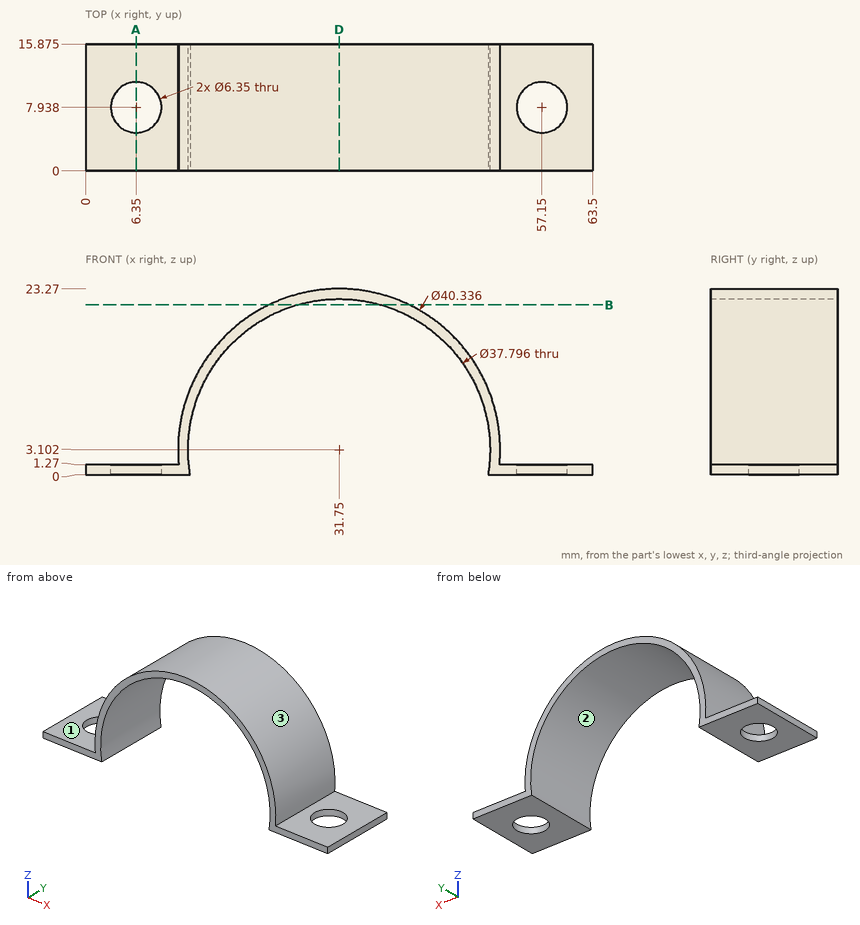
Source: three-view drawing plus pictorial views. Frame: mm from the lowest corner of the part. Coordinates: 2 decimals unless noted, no trailing zeros. Loops run counter-clockwise (first coordinate to the right, second up) from the corner with the lowest first, then second, coordinate; pieces in that order, holes last. Notation, with made-up numbers: (-5.75, 37) -> (29.25, 37) arc R33 cw to (29.25, 76) -> close; hole circle Ø1 at (69, 58). An arc over 180 degrees is marked (long way). Answer in a Markdown table with one row per item. Add a question column.
Q1. Section D-D on x = 31.75. Return the cut outline in (y, z) (1 decimal).
Q2. Section A-A on x = 6.35. Return the cut outline in (y, z) (1 decimal).
Q3. Contact query for flat-ended pins moving along their axis: pin 1 Ø2 at (x, z) = (42.5, 17) entering from +Y; pin 2 Ø6 at (x, y) = (19, 7) entering from +Z; pin 3 Ø6 at (y, z) = (8, 6.5) entering from +X; pin 4 Ø3.5 at (x, y) = (3, 9) entering from +Z. Output: stop coordinate, or through.
Q4. Ray query, line 1 along Y through (x, z) = (6.35, 0.4) (1 decimal); line 2 along Z through (x, y) = (6.5, 1.75); line 3 along Z through (x, y) = (31.75, 5.75). Return the intervals inside material, ascending.
Q5. Pull-direction query (X, two-part tool) for the marked faces 1, 2 and 3; classes: pulls with the +X half, pulls with the -X half, needs draft (parallel to the pull), parting line crosses it, or undercut.
Q6. Section B-B on z = 21.25. Return the cut outline in (x, y) (1 decimal), and give its area (3 significant figures).
Computed values:
| question | item | result |
|---|---|---|
| 1 | outline | (0, 22) -> (15.9, 22) -> (15.9, 23.3) -> (0, 23.3) -> close |
| 2 | outline | (0, 0) -> (4.8, 0) -> (4.8, 1.3) -> (0, 1.3) -> close; (11.1, 0) -> (15.9, 0) -> (15.9, 1.3) -> (11.1, 1.3) -> close |
| 3 | pin 1 | passes through |
| 3 | pin 2 | stops at z = 20.76 |
| 3 | pin 3 | stops at x = 51.91 |
| 3 | pin 4 | stops at z = 1.27 |
| 4 | line 1 | y = 0 to 4.8, 11.1 to 15.9 |
| 4 | line 2 | z = 0 to 1.27 |
| 4 | line 3 | z = 22 to 23.27 |
| 5 | face 1 | needs draft |
| 5 | face 2 | undercut |
| 5 | face 3 | parting line crosses it |
| 6 | outline | (23, 0) -> (26.5, 0) -> (26.5, 15.9) -> (23, 15.9) -> close; (37, 0) -> (40.5, 0) -> (40.5, 15.9) -> (37, 15.9) -> close |
| 6 | area | 112 mm^2 |
